Design review of the part built by this model. Coordinates are the model's own, in mm. Coordinates: 2 decimals unless noted, no trailing zeros.
Q1. Add section A-A on z = -9.5. Give the number of separate pieces and of enclosed holes in the cut face, and give its area (3 significant figures).
Q2. Wall thickness on probe 1 along Y at (x, z) = (-54, -15.5); probe 2 along Y at (x, z) = (-47, -4); probe 3 along Y at (x, z) = (-10.5, -2): over which ranges is each line inside the solid? List them lowest first.
Q3. Draft analysis for pull direction X (two halves, no side actions). For faces 1 (the face through (-63.5, -1, -9)), 2 (the face through (63.5, -1, -9)), 3 (the face through (40.126, 20.672, -9.658)), state which applies: released by +X, released by -X, zero draft, split by the parting line, or undercut.
Q4. For P1, Ø13, axis at x = -10, y = -11.75, coming from the -Z side; P2, Ø1.5, axis at x = -25.5, y = -5.5, coming from the +Z side, all flat-tipped, find the tip position at first contact; note any pin that passes through.
```python
from build123d import *

# Parameters (mm, degrees)
F0_W           = 127
F0_H           = 127
F0_R           = 8.255
F0_R_2         = 3.175
F1_DEPTH       = 19.05
F2_D           = 5.1054
F3_D           = 16.51
F3_CSINK_D     = 18.542
F3_CSINK_ANGLE = 55


with BuildPart() as f1:
    # F0 (on Top) → F1 (new body)
    with BuildSketch(Plane.XY):
        Rectangle(F0_W, F0_H)
        with Locations((-50.0000905, -51.74996)):
            Circle(F0_R, mode=Mode.SUBTRACT)
        with Locations((-30.0000924, -51.74996)):
            Circle(F0_R, mode=Mode.SUBTRACT)
        with Locations((-10.0000943, -51.74996)):
            Circle(F0_R, mode=Mode.SUBTRACT)
        with Locations((-50.0000905, -11.75004)):
            Circle(F0_R, mode=Mode.SUBTRACT)
        with Locations((-30.0000924, -11.75004)):
            Circle(F0_R, mode=Mode.SUBTRACT)
        with Locations((-10.0000943, -11.75004)):
            Circle(F0_R, mode=Mode.SUBTRACT)
        with Locations((9.9999038, -51.74996)):
            Circle(F0_R, mode=Mode.SUBTRACT)
        with Locations((29.9999019, -51.74996)):
            Circle(F0_R, mode=Mode.SUBTRACT)
        with Locations((49.9999, -51.74996)):
            Circle(F0_R, mode=Mode.SUBTRACT)
        with Locations((9.9999038, -11.75004)):
            Circle(F0_R, mode=Mode.SUBTRACT)
        with Locations((29.9999019, -11.75004)):
            Circle(F0_R, mode=Mode.SUBTRACT)
        with Locations((49.9999, -11.75004)):
            Circle(F0_R, mode=Mode.SUBTRACT)
        with Locations((-38.1, 22.225)):
            Circle(F0_R_2, mode=Mode.SUBTRACT)
        with Locations((-12.7, 22.225)):
            Circle(F0_R_2, mode=Mode.SUBTRACT)
        with Locations((12.7, 22.225)):
            Circle(F0_R_2, mode=Mode.SUBTRACT)
        with Locations((38.1, 22.225)):
            Circle(F0_R_2, mode=Mode.SUBTRACT)
        with Locations((-38.1, 22.225)):
            Circle(F0_R_2)
        with Locations((-12.7, 22.225)):
            Circle(F0_R_2)
        with Locations((12.7, 22.225)):
            Circle(F0_R_2)
        with Locations((38.1, 22.225)):
            Circle(F0_R_2)
        with Locations((49.9999, -11.75004)):
            Circle(F0_R)
        with Locations((29.9999019, -11.75004)):
            Circle(F0_R)
        with Locations((9.9999038, -11.75004)):
            Circle(F0_R)
        with Locations((-10.0000943, -11.75004)):
            Circle(F0_R)
        with Locations((-30.0000924, -11.75004)):
            Circle(F0_R)
        with Locations((-50.0000905, -11.75004)):
            Circle(F0_R)
        with Locations((-50.0000905, -51.74996)):
            Circle(F0_R)
        with Locations((-30.0000924, -51.74996)):
            Circle(F0_R)
        with Locations((-10.0000943, -51.74996)):
            Circle(F0_R)
        with Locations((9.9999038, -51.74996)):
            Circle(F0_R)
        with Locations((29.9999019, -51.74996)):
            Circle(F0_R)
        with Locations((49.9999, -51.74996)):
            Circle(F0_R)
    extrude(amount=-F1_DEPTH)

    # F2 (through all)
    with Locations(Plane.XY):
        with Locations((-38.1, 22.225), (-12.7, 22.225), (12.7, 22.225), (38.1, 22.225)):
            Hole(F2_D / 2)

    # F3 (through all)
    with Locations(Plane.XY):
        with Locations((-50.0000905, -11.75004), (-30.0000924, -11.75004), (-10.0000943, -11.75004), (9.9999038, -11.75004), (29.9999019, -11.75004), (49.9999, -11.75004), (49.9999, -51.74996), (29.9999019, -51.74996), (9.9999038, -51.74996), (-10.0000943, -51.74996), (-30.0000924, -51.74996), (-50.0000905, -51.74996)):
            CounterSinkHole(F3_D / 2, F3_CSINK_D / 2, counter_sink_angle=F3_CSINK_ANGLE)


solid = f1.part
```
Entries:
1. separate pieces: 1
1. enclosed holes: 16
1. area: 13,500 mm2
2. probe 1: y = -63.5 to -58.97, -44.53 to -18.97, -4.53 to 63.5
2. probe 2: y = -63.5 to -59.44, -44.06 to -19.44, -4.06 to 63.5
2. probe 3: y = -63.5 to -59.99, -43.51 to -19.99, -3.51 to 20.93, 23.52 to 63.5
3. face 1: released by -X
3. face 2: released by +X
3. face 3: undercut
4. P1: passes through
4. P2: stops at z = -1.57
